For this review, take the finished solid that the model builds, in its own axes (mm). A direction names the side the tool comes from. Coordinates: 2 decimals unless noted, no trailing zeros. Order: outer loops, then holes, each group sorted by start corner. A loop starts at its lowest first (then second) coordinate and runs counter-clockwise, first axis right, second up. Notation, with made-up numbers: (65.25, 40) - (109.25, 40) arc R27 ccw to (109.25, 58) - close; hole circle Ø8 at (30, 56). An arc over 180 degrees is marked (long way). One line per item, written item: value. Start each with the question number.
(1) Mouldability with a two-part tool opening along X and no side actions: class faces 6 (the flat face through (-19, 45, 32)), 7 (the cylindrical face through (4.036, -30.736, 146.056)), 8 (the flat face through (20, -25, 66)) as released by +X, released by -X, zero draft, split by the parting line, or undercut.
(2) Consider section A-A on y = 0. Write out the cut boundary in (x, z), then the cut area to 3 significant figures.
(3) Consider section D-D on x = 0. Count the separate pieces of the cut face and the enclosed holes in it, then the cut area to 3 significant figures.
(4) Clearance check with flat-ended pins moving along their axes: pin 1 (12 mm diameter, centred on y = -42, z = 94.5, fed in from +X); pin 2 (12 mm diameter, centred on y = -14.5, z = 77.5, fed in from +X); pin 3 (2 mm diameter, centred on x = 6, z = 119, fed in from +Y). State where each tip first meets the part, or that it passes through.
(5) To check wall thickness, follow line 1 along Y through (x, z) = (-53, 78.5); line 2 along Z through (x, y) = (0, -44.5); line 3 along X through (y, z) = (-48.5, 60). State the ranges of each line that lie inside material, in increasing order.
(6) Consider section C-C on z = 94. Write out the cut boundary in (x, y), then the cut area to 3 significant figures.
(7) For faces 1 (the cylindrical face through (-6.503, -49.93, 89.287)), 2 (the flat face through (14, 30, 31)), 3 (the cylindrical face through (-67.08, 0.44, 56.2)), 4 (the flat face through (1, 31, 0)), 5 (the cylindrical face through (-6.503, 49.93, 89.287)), list the 3-axis set-ups (+Z, -Z, +X, -X, +Y, -Y) from which the entire face can be reached by the end or side of a thin tool; tool diameter is ignored.
```python
from build123d import *

# Parameters (mm, degrees)
EXTRUDE_1_DEPTH     = 120
CUT_EXTRUDE_1_DEPTH = 114
SKETCH_5_R          = 20
CUT_EXTRUDE_3_DEPTH = 91
EXTRUDE_START       = 25
SKETCH_6_R          = 30
SKETCH_6_R_2        = 20
EXTRUDE_2_DEPTH     = 30
FILLET_2_R          = 5
FILLET_3_R          = 5


with BuildPart() as part:
    # 草图1 → 凸台-拉伸1 (new body)
    with BuildSketch(Plane.XY):
        with BuildLine():
            Line((-80, 45), (80, 45))
            ThreePointArc((80, 45), (91.787798753, 0), (80, -45))
            Line((80, -45), (-80, -45))
            ThreePointArc((-80, -45), (-91.787798753, 0), (-80, 45))
        make_face()
    extrude(amount=EXTRUDE_1_DEPTH)

    # 草图3 → 切除-拉伸1 (cut)
    with BuildSketch(Plane(origin=(0, 0, 0), x_dir=(-1, 0, 0), z_dir=(0, 0, -1))):
        with BuildLine():
            Line((-60, 30), (60, 30))
            ThreePointArc((60, 30), (67.082039325, 0), (60, -30))
            Line((60, -30), (-60, -30))
            ThreePointArc((-60, -30), (-67.082039325, 0), (-60, 30))
        make_face()
    extrude(amount=-CUT_EXTRUDE_1_DEPTH, mode=Mode.SUBTRACT)

    # 草图5 → 切除-拉伸3 (cut, through all)
    with BuildSketch(Plane.XZ.offset(45)):
        with Locations((0, 60)):
            Circle(SKETCH_5_R)
    extrude(amount=-CUT_EXTRUDE_3_DEPTH, mode=Mode.SUBTRACT)

    # 草图6 → 凸台-拉伸2 (add)
    with BuildSketch(Plane(origin=(0, 0, 0), x_dir=(1, 0, 0), z_dir=(0, 1, 0)).offset(EXTRUDE_START)):
        with Locations((0, -60)):
            Circle(SKETCH_6_R)
        with Locations((0, -60)):
            Circle(SKETCH_6_R_2, mode=Mode.SUBTRACT)
    extrude_2 = extrude(amount=EXTRUDE_2_DEPTH)

    # 镜向1: 凸台-拉伸2 across plane
    add(extrude_2.mirror(Plane.ZX))

    # 草图9 → 旋转1 (revolve)
    with BuildSketch(Plane(origin=(0, 0, 0), x_dir=(1, 0, 0), z_dir=(0, 1, 0))):
        Polygon((0, -120), (-25, -120), (-25, -142), (-31, -142), (-31, -150), (0, -150), align=None)
    revolve(axis=Axis((0, 0, -35.705886154), (0, 0, 1)))

    # 圆角2
    fillet_2_edges = [part.edges().sort_by_distance(p)[0] for p in [
        (25, 0, 120),
    ]]
    fillet(fillet_2_edges, radius=FILLET_2_R)

    # 圆角3
    fillet_3_edges = [part.edges().sort_by_distance(p)[0] for p in [
        (25, 0, 142),
    ]]
    fillet(fillet_3_edges, radius=FILLET_3_R)

    # 草图10 → 切除-旋转1 (revolve, cut)
    with BuildSketch(Plane(origin=(0, 0, 0), x_dir=(1, 0, 0), z_dir=(0, 1, 0))):
        Polygon((0, -150), (-15, -150), (-12.5, -105), (0, -105), align=None)
    revolve(axis=Axis((0, 0, 161.939554525), (0, 0, -1)), mode=Mode.SUBTRACT)


solid = part.part
```
Geometry check:
1. face 6: zero draft
1. face 7: split by the parting line
1. face 8: undercut
2. outline: (-91.79, 0) - (-67.08, 0) - (-67.08, 114) - (-13, 114) - (-15, 150) - (-31, 150) - (-31, 142) - (-30, 142) arc R5 cw to (-25, 137) - (-25, 125) arc R5 cw to (-30, 120) - (-91.79, 120) - close; (13, 114) - (67.08, 114) - (67.08, 0) - (91.79, 0) - (91.79, 120) - (30, 120) arc R5 cw to (25, 125) - (25, 137) arc R5 cw to (30, 142) - (31, 142) - (31, 150) - (15, 150) - close
2. area: 7,340 mm^2
3. separate pieces: 4
3. enclosed holes: 0
3. area: 3,970 mm^2
4. pin 1: stops at x = 84.43
4. pin 2: stops at x = 91.39
4. pin 3: stops at y = 45
5. line 1: y = -45 to -30, 30 to 45
5. line 2: z = 0 to 40, 80 to 120
5. line 3: x = -30 to -20, 20 to 30
6. outline: (-80, -45) - (80, -45) arc R91.79 ccw to (80, 45) - (-80, 45) arc R91.79 ccw to start; hole (-60, -30) - (60, -30) arc R67.08 ccw to (60, 30) - (-60, 30) arc R67.08 ccw to start
6. area: 8,060 mm^2
7. face 1: -Y
7. face 2: none
7. face 3: -Z
7. face 4: -Z, +X, -X, +Y, -Y
7. face 5: +Y
